Build history of the part. All positions in model axes, mm. Give positions to 0.01 mm unless a question says otherwise; leave off trailing zeros. Loops run counter-clockwise (first coordinate to the right, second up) from the corner with the lowest first, then second, coordinate; pieces in that order, holes last. Notation, with made-up numbers: (17.5, -32.5) - (44.5, -32.5) arc R19 cw to (44.5, -25.5) - close; hole circle Ø10 at (2, 18.5). An arc over 180 degrees is marked (long way). Return JSON: item names as keys, results as strings. Group by question number.
1) Slice it at A-A (y = 18.5). List the corners of the cut face in (x, z).
2) Drop flat-ended pins along their axis: pin 1 (4 mm diameter, centred on x = 3.5, z = 19.5, fed in from -Y); pin 2 (5 mm diameter, centred on x = -8, z = -10.5, fed in from +Y); pin 3 (4 mm diameter, centred on y = 7, z = 14.5, fed in from +X); pin 4 (3 mm diameter, centred on x = -37.5, z = -19.5, fed in from -Y). Give the stop position or say it passes through.
3) Drill centre lines: probe 1 along Y at (x, z) = (-19, -13); probe 2 along Z at (x, y) = (0, 7.5); probe 3 along Z at (x, y) = (-17.5, 23). Where is each one in solid material? Low to high. Write a range as from..to.
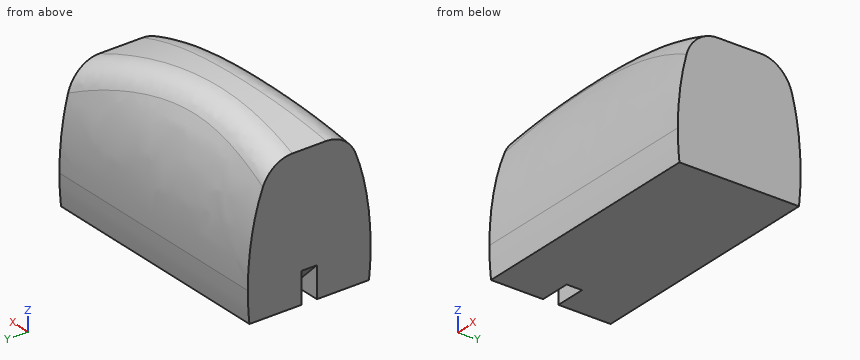
Autodesk Inventor part; units mm, degrees
ref_plane "YZ Plane" through (0, 0, 0) normal (1, 0, 0) x (0, 1, 0)
ref_plane "XZ Plane" through (0, 0, 0) normal (0, 1, 0) x (-1, 0, 0)
ref_plane "XY Plane" through (0, 0, 0) normal (0, 0, 1) x (1, 0, 0)
sketch "スケッチ1" plane through (0, 0, 0) normal (0, 1, 0) x (-1, 0, 0)
  line L0 (-40, 25) -> (40, 25)
  line L1 (40, 25) -> (40, -25)
  line L2 (40, -25) -> (-40, -25)
  line L3 (-40, -25) -> (-40, 25)
  line L4 (-40, 25) -> (40, -25) construction
  line L5 (40, 25) -> (-40, -25) construction
  circle A0 centre (7, -100) radius 125
  line L6 (40, -15) -> (30, -25)
  point P0 (0, 0)
  point P1 (40, 20.5653)
  point P2 (-40, 15.8275)
  dimension "d0" = 80
  dimension "d1" = 50
  dimension "d2" = 7
  dimension "d3" = 250
  dimension "d6" = 10
  dimension "d7" = 10
extrude "押し出し1" add sketch "スケッチ1" along normal blind 40 contours A0 L1 L6 L2 L3 | L1 L2 L6
ref_plane "作業平面1" through (0, 17.5, 0) normal (0, 1, 0) x (1, 0, 0)
sketch "スケッチ2" plane through (0, 17.5, 0) normal (0, 1, 0) x (1, 0, 0)
  line L0 (40, -15.8275) -> (40, 25)
  line L1 (40, 25) -> (-40, 25)
  line L2 (-40, 25) -> (-40, -20.5653)
  arc A0 (-40, -20.5653) -> (40, -15.8275) centre (-7, 100) ccw
  line L3 (-40, 15) -> (-30, 25)
  line L4 (40, 25) -> (-40, 25)
  point P0 (0, 0)
  dimension "d11" = 10
  dimension "d12" = 45
extrude "押し出し2" cut sketch "スケッチ2" along normal blind 5 contours L3 L2 L1
sketch "スケッチ3" plane through (40, 0, 15.8275) normal (1, 0, 0) x (0, 0, -1)
  line L0 (-9.1725, 0) -> (-9.1725, 40)
  line L1 (0, 0) -> (40.8275, 0)
  line L2 (0, 0) -> (-9.1725, 0)
  line L3 (0, 40) -> (-9.1725, 40)
  line L4 (0, 40) -> (40.8275, 40)
  line L5 (40.8275, 0) -> (40.8275, 40)
  line L6 (40.8275, 20) -> (-7.81, 20)
  ellipse E0 centre (30.8275, 20) end of major axis (-13.1725, 20) minor radius 20
  point P0 (15.8275, 0)
  point P1 (-4.7379, 0)
  point P2 (-4.7379, 40)
  point P3 (-9.1725, 28.332)
  point P4 (30.8275, 40)
  point P5 (40.8275, 39.4766)
  point P6 (30.8275, 0)
  point P7 (-9.1725, 11.668)
  point P8 (40.8275, 0.5234)
  dimension "d15" = 44
  dimension "d16" = 10
extrude "押し出し3" cut sketch "スケッチ3" against normal through all contours L0 E0 L1 L2 | L0 L3 L4 E0 | E0 L5 L1 | L4 L5 E0
fillet "フィレット2" radius 10 4 edges at (16.84, 9.6918, 22.7056) (-23.6437, 10.6425, 23.887) (16.84, 30.3082, 22.7056) (-23.6437, 29.3575, 23.887)
Results:
{
 "1": {"outline": "(-40, -15) - (-30, -25) - (40, -25) - (40, 15.83) arc R125 ccw to (-40, 20.57) - close"},
 "2": {"pin 1": "y = 6.52", "pin 2": "y = 39.98", "pin 3": "x = 40", "pin 4": "y = 0.05"},
 "3": {"probe 1": "0.02..39.98", "probe 2": "-25..19.35", "probe 3": "-25..24.56"}
}
